Read the model definition and answer for the solid it produces. Units are mm, in the model's axes. A direction names the side the tool comes from. Round coordinates to 2 decimals unless told otherwise and drop trailing zeros. Order: outer loops, then holes, each group sorted by start corner. A loop starts at its lowest first (then second) coordinate and runs counter-clockwise, first axis right, second up. Notation, with made-up numbers: (-2.5, -0.75) - (32.5, -0.75) arc R18 cw to (32.5, 28.25) - close; hole circle Ø11 at (2, 30). An arc over 180 degrees is marked (long way). Put each result on its own line as item: value. Start each with the question number.
Q1. Which of the six approach directions +Z, -Z, +X, -X, +Y, -Y give full straight-line access (tool end or side, diameter ignored) to faces 1 (the face through (11.056, -7.907, 1.756)), 2 (the face through (-8.8, 7, -3)), 3 (the face through (-11, -7, 11))?
Q2. For a pull along Y with two mould halves and no side action, classify faces 4 (the face through (0.154, 11.923, 3.755)), 5 (the face through (11, -7, -11)), 6 (the face through (-11.056, 7.907, 1.756)) as pulls with the +Y half, pulls with the -Y half, needs draft (parallel to the pull), parting line crosses it, or undercut.
Q3. Find the intervals of material crossed by line 1 along X through (y, z) = (-13, 4.5); line 2 along Z through (x, y) = (0.25, 0); line 3 along Z through (x, y) = (-10.55, 0), in increasing order. Write a range as from..to.
Q4. Section A-A on x = 11.75 is taken. Give the vertices of the cut face in (y, z), then the cut area to 3 significant figures.
Q5. Each of these flat-tipped pins is pushed along its axis until it touches: pin 1 Ø14.5 at (y, z) = (0, 0) entering from +X; pin 2 Ø6 at (x, z) = (9.5, 4) entering from +Y; pin 3 Ø8 at (x, z) = (-4, 12) entering from +Y. Where does it stop, or does it pass through?
Q6. Section B-B on x = 1.5 is taken. Give the vertices of the cut face in (y, z).
Solid Edge part; units mm, degrees
sketch "Sketch1" plane through (0, 0, 0) normal (1, 0, 0) x (0, 1, 0)
  circle A0 centre (0, 0) radius 12.5
extrude "Extrusionsausprägung_15" add sketch "Sketch1" along normal mid plane 22
sketch "Sketch2" plane through (-11, 0, 0) normal (-1, 0, 0) x (0, -1, 0)
  circle A0 centre (0, 0) radius 15.5
extrude "Extrusionsausprägung_16" add sketch "Sketch2" along normal blind 3
chamfer "Fase_9" distance 1.5 distance2 1 1 edges at (-11, 15.5, 0) measured on face at (-13.47, -8.5776, 12.9103)
sketch "Sketch3" plane through (-14, 0, 0) normal (-1, 0, 0) x (0, 0, -1)
  circle A0 centre (0, 0) radius 8.1
extrude "Extrusionsausschnitt_23" cut sketch "Sketch3" against normal blind 5.2
chamfer "Fase_10" distance 0.75 angle 45 1 edges at (-14, 0, 8.1)
chamfer "Fase_11" distance 0.5 angle 45 1 edges at (-14, 15.5, 0)
mirror "Mirror1" about plane through (0, 0, 0) normal (1, 0, 0) of "Extrusionsausprägung_16", "Fase_9", "Extrusionsausschnitt_23", "Fase_10", "Fase_11"
sketch "Sketch4" plane through (8.8, 0, 0) normal (1, 0, 0) x (0, 0, 1)
  circle A0 centre (0, 0) radius 5.15
extrude "Extrusionsausschnitt_24" cut sketch "Sketch4" against normal blind 20
chamfer "Fase_12" distance 2 angle 45 2 edges at (8.8, 0, -5.15) (-8.8, -5.15, 0)
Findings:
1. face 1: +X
1. face 2: -X
1. face 3: none
2. face 4: parting line crosses it
2. face 5: needs draft
2. face 6: undercut
3. line 1: -14..-11, 11..14
3. line 2: -12.5..-5.15, 5.15..12.5
3. line 3: -12.5..-8.1, 8.1..12.5
4. outline: circle Ø30 at (0, 0); hole circle Ø16.2 at (0, 0)
4. area: 501 mm2
5. pin 1: x = 8.8
5. pin 2: y = 15.09
5. pin 3: y = 9.6
6. outline: circle Ø25 at (0, 0); hole circle Ø10.3 at (0, 0)
